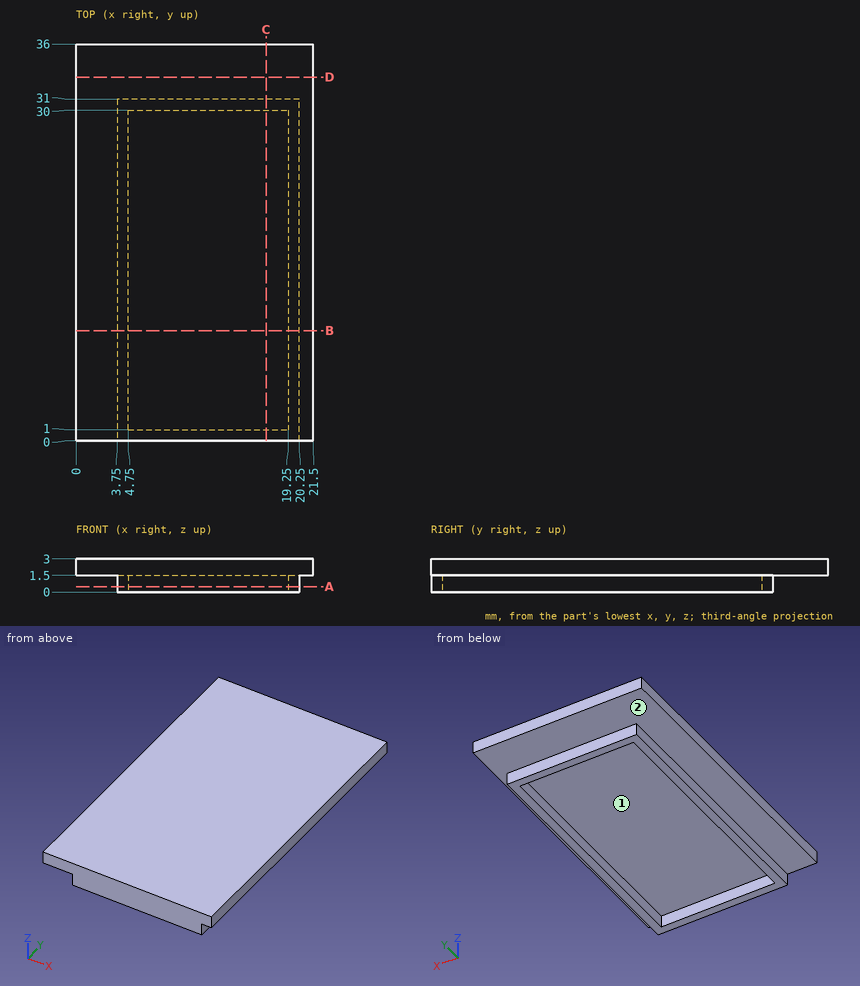
Geometry: see drawing. Coordinates: mm, zero at the bounding-box minimum. Give positions to 0.01 mm unless a question says otherwise; leave off trailing zeros. Loops run counter-clockwise (first coordinate to the right, second up) from the corner with the lowest first, then second, coordinate; pieces in that order, holes last. Notation, with made-up numbers: (75.25, -30.75) - (82.25, -30.75) arc R25 ccw to (82.25, -7.75) - close; hole circle Ø9 at (16.25, -22). An arc over 180 degrees is marked (long way). Use CSV: the item, a comma, the result in double quotes. Start each with the question number.
1. Draft query along X for the marked faces 1 and 2. Return one class per face: +X half, -X half, draft (parallel to the pull), parting line (faces both ways), or undercut.
2. Pin query (flat end, axial travel): pin 1 (4.5 mm diameter, centred on x = 8.5, y = 11, fed in from -Z); pin 2 (0.8 mm diameter, centred on y = 20.5, z = 1, fed in from +X); pin 3 (1.2 mm diameter, centred on x = 14, z = 0.5, fed in from +Y). Return the tip coordinate at first contact, or that it passes through.
3. Section D-D (y = 33). Output: boundary loops of the cut face in (x, z).
4. Section B-B (y = 10). Output: boundary loops of the cut face in (x, z), then the cut area to 4 significant figures.
5. Section C-C (x = 17.25). Output: boundary loops of the cut face in (y, z), then the cut area to 3 significant figures.
6. Ray query, L1, parallel to X at y = 6, z = 1.2; L2, parallel to Y at x = 11.5, z = 0.9; L3, parallel to Z at x = 18.5, y = 32. Return the intervals inside material, ascending.
7. Section A-A (z = 0.5). Output: boundary loops of the cut face in (x, y), then the cut area to 3 significant figures.
Response:
1,face 1,"undercut"
1,face 2,"draft"
2,pin 1,"z = 1.5"
2,pin 2,"x = 20.25"
2,pin 3,"y = 31"
3,outline,"(0, 1.5) - (21.5, 1.5) - (21.5, 3) - (0, 3) - close"
4,outline,"(0, 1.5) - (3.75, 1.5) - (3.75, 0) - (4.75, 0) - (4.75, 1.5) - (19.25, 1.5) - (19.25, 0) - (20.25, 0) - (20.25, 1.5) - (21.5, 1.5) - (21.5, 3) - (0, 3) - close"
4,area,"35.25 mm²"
5,outline,"(0, 0) - (1, 0) - (1, 1.5) - (30, 1.5) - (30, 0) - (31, 0) - (31, 1.5) - (36, 1.5) - (36, 3) - (0, 3) - close"
5,area,"57.0 mm²"
6,L1,"3.75 to 4.75, 19.25 to 20.25"
6,L2,"0 to 1, 30 to 31"
6,L3,"1.5 to 3"
7,outline,"(3.75, 0) - (20.25, 0) - (20.25, 31) - (3.75, 31) - close; hole (4.75, 1) - (19.25, 1) - (19.25, 30) - (4.75, 30) - close"
7,area,"91.0 mm²"
